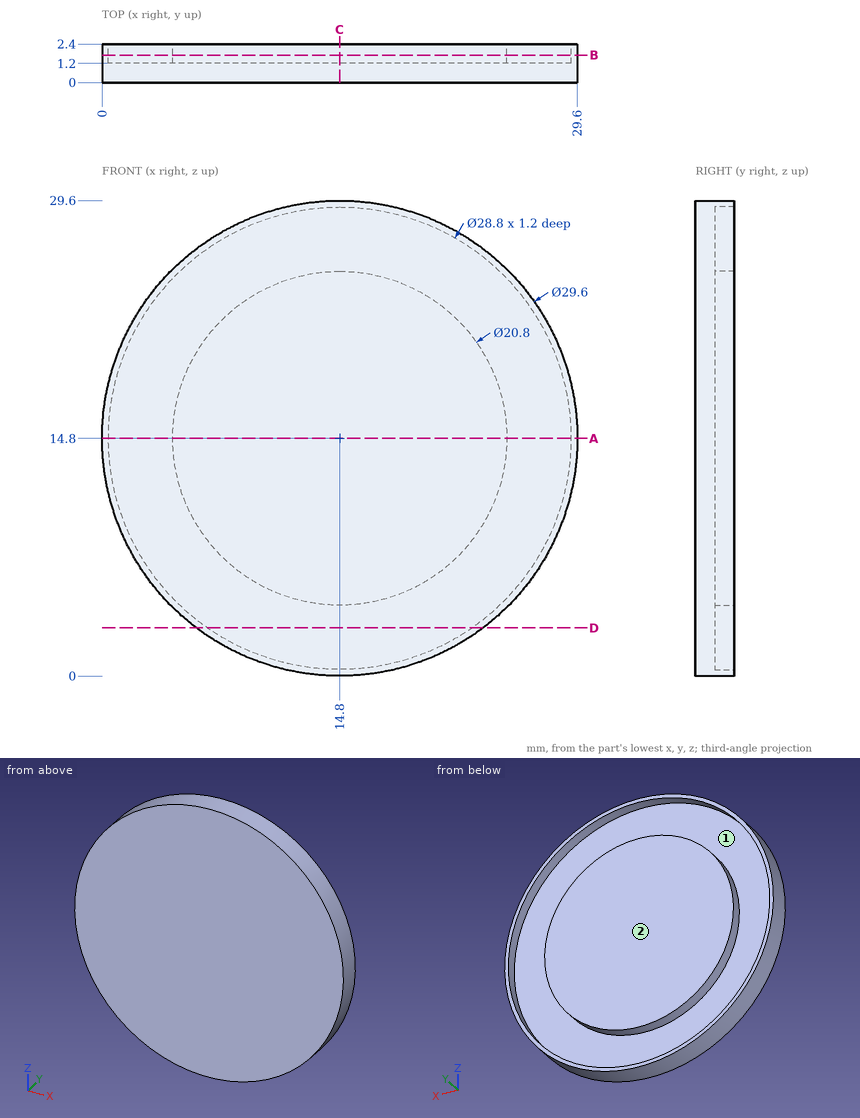
Can you work these out from the drawing? Everything is in mm from the part's minimum corner. Round coordinates to 2 decimals unless told otherwise and drop trailing zeros. Loops run counter-clockwise (first coordinate to the right, second up) from the corner with the lowest first, then second, coordinate; pieces in that order, holes last. Notation, with made-up numbers: (75.25, -29) -> (110.25, -29) arc R30 ccw to (110.25, -6) -> close; hole circle Ø3 at (42, -33.75). An arc over 180 degrees is marked (long way). One line per question, with ' | ' between items.
(1) If we section it at A-A on z = 14.8: List the corners of the cut face in (x, y) for me.
Model answer:
outline: (0, 0) -> (29.6, 0) -> (29.6, 2.4) -> (29.2, 2.4) -> (29.2, 1.2) -> (25.2, 1.2) -> (25.2, 2.4) -> (4.4, 2.4) -> (4.4, 1.2) -> (0.4, 1.2) -> (0.4, 2.4) -> (0, 2.4) -> close
(2) If we section it at D-D on z = 3: List the corners of the cut face in (x, y) for me.
Model answer:
outline: (5.87, 0) -> (23.73, 0) -> (23.73, 2.4) -> (23.05, 2.4) -> (23.05, 1.2) -> (6.55, 1.2) -> (6.55, 2.4) -> (5.87, 2.4) -> close
(3) If we section it at B-B on y = 1.7: List the corners of the cut face in (x, z) for me, and give its area (3 significant figures).
Model answer:
outline: circle Ø29.6 at (14.8, 14.8); circle Ø20.8 at (14.8, 14.8); hole circle Ø28.8 at (14.8, 14.8) | area: 376 mm^2
(4) Thinking about a two-plate mould opening in X: for the marked faces 1 and 2, which applies, released by +X, released by -X, zero draft, split by the parting line, or undercut?
Model answer:
face 1: undercut | face 2: zero draft
(5) If I drill on probe 1 along X at (y, z) = (1.65, 14.8); probe 2 along Z at (x, y) = (18.25, 1.4), over which ranges is the centre line in solid material (lowest first)?
Model answer:
probe 1: x = 0 to 0.4, 4.4 to 25.2, 29.2 to 29.6 | probe 2: z = 0.41 to 0.82, 4.99 to 24.61, 28.78 to 29.19
(6) For pin 1 Ø1 at (x, y) = (21.5, 1.5) entering from +Z, with a flat end and sliding along its axis, tell me the tip position at first contact or that it passes through.
Model answer:
pin 1: stops at z = 28.24
(7) If we section it at C-C on x = 14.8: List the corners of the cut face in (y, z) for me.
Model answer:
outline: (0, 0) -> (2.4, 0) -> (2.4, 0.4) -> (1.2, 0.4) -> (1.2, 4.4) -> (2.4, 4.4) -> (2.4, 25.2) -> (1.2, 25.2) -> (1.2, 29.2) -> (2.4, 29.2) -> (2.4, 29.6) -> (0, 29.6) -> close
